The drawing under review shows one solid part. Ordinate dimensions are in mm from its lowest x, y, z. A direction names the side the tool comes from. Give positions to 0.01 mm unless a question says otherwise; leave off trailing zeros. Loops run counter-clockwise (first coordinate to the right, second up) from the corner with the lowest first, then second, coordinate; pieces in that order, holes last. Notation, with made-up numbers: (0.5, -8.75) - (37.5, -8.75) arc R15 cw to (37.5, 5.25) - close; hole circle Ø8 at (-13, -3.5). An arc over 180 degrees is marked (long way). Answer as CSV lines item,"result".
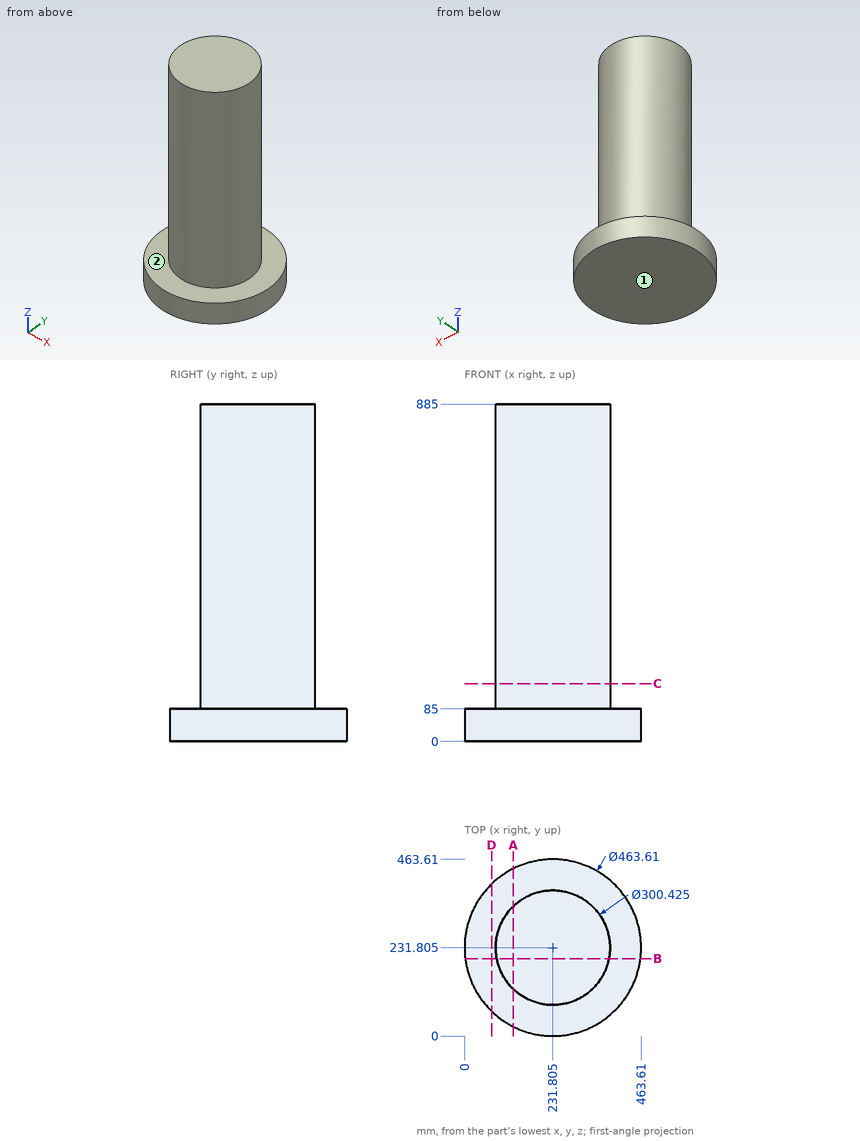
1) Insertion check: P1, Ø2, axis at y = 106.5, z = 405, coming from the +X side; P2, Ø6, axis at x = 210, z = 567, coming from the +Y side; P3, Ø5, axis at y = 333, z = 296, coming from the +X side (1 decimal); P4, Ø6, axis at x = 380, y = 96, coming from the -Z side. Each pin has a flat end and moves straight along its axis. Give the tip position at first contact, or say it passes through.
From the geometry:
P1,"stops at x = 316.14"
P2,"stops at y = 380.84"
P3,"stops at x = 345"
P4,"stops at z = 0"
2) Consider section A-A on x = 128. Write out the cut boundary in (y, z).
From the geometry:
outline,"(24.54, 0) - (439.07, 0) - (439.07, 85) - (340.38, 85) - (340.38, 885) - (123.23, 885) - (123.23, 85) - (24.54, 85) - close"
3) Consider section B-B on y = 203. Write out the cut boundary in (x, z).
From the geometry:
outline,"(1.8, 0) - (461.81, 0) - (461.81, 85) - (379.23, 85) - (379.23, 885) - (84.38, 885) - (84.38, 85) - (1.8, 85) - close"
4) Consider section D-D on x = 71. Write out the cut boundary in (y, z) (1 decimal).
From the geometry:
outline,"(64.8, 0) - (398.8, 0) - (398.8, 85) - (64.8, 85) - close"
5) Wall thickness on line 1 (Z direction, x = 404.5, y = 266); line 2 (Y direction, x = 231, z = 643) (1 decimal); line 3 (X direction, y = 218, z = 413.5): over which ranges is each line inside the solid? List them lowest first. Write a range as from..to.
From the geometry:
line 1,"z = 0..85"
line 2,"y = 81.6..382"
line 3,"x = 82.23..381.38"
6) Machinability: for the marked faces 1 and 2, which of the approach directions +Z, -Z, +X, -X, +Y, -Y give a long, thin tool a straight path to every point of the face, cutting with its end or side? Answer none if there is none.
From the geometry:
face 1,"-Z, +X, -X, +Y, -Y"
face 2,"+Z"
7) Consider section C-C on z = 151.5. Write out the cut boundary in (x, y) (1 decimal).
From the geometry:
outline,"circle Ø300.4 at (231.8, 231.8)"
